For this review, take the finished solid that the model builds, in its own axes (mm). A direction names the side the tool comes from. Coordinates: 2 decimals unless noted, no trailing zeros. Write each loop counter-clockwise with the first axis right and the second up, starting at its lowest first coordinate (ties: lowest second). Pieces come first, ordered by that corner, then holes.
```python
from build123d import *

# Parameters (mm, degrees)
SKETCH2_R           = 1
BOSS_EXTRUDE1_DEPTH = 0.375
CHAMFER1_SIZE       = 0.25
CHAMFER2_SIZE       = 0.5
FILLET1_R           = 0.25


with BuildPart() as part:
    # Sketch1 → Revolve1 (revolve)
    with BuildSketch(Plane.XY):
        with BuildLine():
            Line((-2, 0), (-5.25, 0))
            Line((-5.25, 0), (-5.25, -3))
            Line((-5.25, -3), (-4, -3))
            Line((-4, -3), (-4, -12))
            Line((-4, -12), (-3.34, -12))
            Line((-3.34, -12), (-3.34, -16.5))
            ThreePointArc((-3.34, -16.5), (-3.193553391, -16.853553391), (-2.84, -17))
            Line((-2.84, -17), (-2.5, -17))
            Line((-2.5, -17), (-2.5, -20))
            Line((-2.5, -20), (0, -20))
            Line((0, -20), (0, -8))
            Line((0, -8), (-2, -8))
            Line((-2, -8), (-2, 0))
        make_face()
    revolve(axis=Axis((0, -20, 0), (0, -1, 0)))

    # Sketch2 → Boss-Extrude1 (add, symmetric)
    with BuildSketch(Plane.XY):
        with BuildLine():
            Line((-2.4, -20), (-2.4, -27.8))
            ThreePointArc((-2.4, -27.8), (-2.253553391, -28.153553391), (-1.9, -28.3))
            Line((-1.9, -28.3), (1.9, -28.3))
            ThreePointArc((1.9, -28.3), (2.253553391, -28.153553391), (2.4, -27.8))
            Line((2.4, -27.8), (2.4, -20))
            Line((2.4, -20), (-2.4, -20))
        make_face()
        with Locations((0, -24.15)):
            Circle(SKETCH2_R, mode=Mode.SUBTRACT)
    extrude(amount=BOSS_EXTRUDE1_DEPTH, both=True)

    # Chamfer1
    # the kernel refuses this chamfer: 0.25 mm, written as the material it takes off along each edge
    with BuildSketch(Plane(origin=(0, -20, 0), x_dir=(-1, 0, 0), z_dir=(0, 0, 1))) as chamfer1_piece_1_section:
        Polygon((2.5 - CHAMFER1_SIZE, 0), (2.5, -CHAMFER1_SIZE), (2.5, 0), align=None)
    chamfer1_piece_1 = revolve(axis=Axis((0, -20, 0), (0, -1, 0)), mode=Mode.PRIVATE)
    chamfer1_piece_1 = split(chamfer1_piece_1, bisect_by=Plane(origin=(-2.4, -19.896022541, 0), z_dir=(-1, 0, 0)), keep=Keep.TOP, mode=Mode.PRIVATE)
    add(chamfer1_piece_1, mode=Mode.SUBTRACT)
    with BuildSketch(Plane(origin=(0, -20, 0), x_dir=(-1, 0, 0), z_dir=(0, 0, 1))) as chamfer1_piece_2_section:
        Polygon((2.5 - CHAMFER1_SIZE, 0), (2.5, -CHAMFER1_SIZE), (2.5, 0), align=None)
    chamfer1_piece_2 = revolve(axis=Axis((0, -20, 0), (0, -1, 0)), mode=Mode.PRIVATE)
    chamfer1_piece_2 = split(chamfer1_piece_2, bisect_by=Plane(origin=(-7e-09, -19.879189064, -0.375), z_dir=(0, 0, -1)), keep=Keep.TOP, mode=Mode.PRIVATE)
    add(chamfer1_piece_2, mode=Mode.SUBTRACT)
    with BuildSketch(Plane(origin=(0, -20, 0), x_dir=(-1, 0, 0), z_dir=(0, 0, 1))) as chamfer1_piece_3_section:
        Polygon((2.5 - CHAMFER1_SIZE, 0), (2.5, -CHAMFER1_SIZE), (2.5, 0), align=None)
    chamfer1_piece_3 = revolve(axis=Axis((0, -20, 0), (0, -1, 0)), mode=Mode.PRIVATE)
    chamfer1_piece_3 = split(chamfer1_piece_3, bisect_by=Plane(origin=(-7e-09, -19.879189064, 0.375), z_dir=(0, 0, 1)), keep=Keep.TOP, mode=Mode.PRIVATE)
    add(chamfer1_piece_3, mode=Mode.SUBTRACT)
    with BuildSketch(Plane(origin=(0, -20, 0), x_dir=(-1, 0, 0), z_dir=(0, 0, 1))) as chamfer1_piece_4_section:
        Polygon((2.5 - CHAMFER1_SIZE, 0), (2.5, -CHAMFER1_SIZE), (2.5, 0), align=None)
    chamfer1_piece_4 = revolve(axis=Axis((0, -20, 0), (0, -1, 0)), mode=Mode.PRIVATE)
    chamfer1_piece_4 = split(chamfer1_piece_4, bisect_by=Plane(origin=(2.4, -19.896022542, 0), z_dir=(1, 0, 0)), keep=Keep.TOP, mode=Mode.PRIVATE)
    add(chamfer1_piece_4, mode=Mode.SUBTRACT)

    # Chamfer2
    chamfer2_edges = [part.edges().sort_by_distance(p)[0] for p in [
        (4, -12, 0),
    ]]
    chamfer(chamfer2_edges, length=CHAMFER2_SIZE)

    # Fillet1
    fillet1_edges = [part.edges().sort_by_distance(p)[0] for p in [
        (2, -8, 0),
        (5.25, -3, 0),
        (5.25, 0, 0),
        (2, 0, 0),
    ]]
    fillet(fillet1_edges, radius=FILLET1_R)


solid = part.part
```
Q1. Tool access review of faces 1 (the cylindrical face through (0.867, -7.31, 3.905)), 2 (the flat face through (0, -20, 1)), 3 (the flat face through (0, -8, 0)): name each direction out of +Z, -Z, +X, -X, +Y, -Y from which nothing blocks a thin tool from reaching the whole face with its end or side.
Ans:
face 1: -Y
face 2: +Z, +X, -X, -Y
face 3: +Y
Q2. Draft analysis for pull direction X (two halves, no side actions). For faces 4 (the cylindrical face through (0.54, -18.39, 2.44)), 5 (the cylindrical face through (0, -4, 2)), 6 (the flat face through (1, -23, -0.375)), state which applies: +X half, -X half, draft (parallel to the pull), parting line (faces both ways), or undercut.
Ans:
face 4: parting line
face 5: undercut
face 6: draft
Q3. For probe 1 along Y at (x, z) = (0, -0.2); probe 2 along X at (y, z) = (-5.5, 0); probe 3 along X at (y, z) = (-8.5, 0), list the stretches that pass through material, from the lowest coordinate up.
Ans:
probe 1: y = -28.3 to -25.15, -23.15 to -8
probe 2: x = -4 to -2, 2 to 4
probe 3: x = -4 to 4
Q4. Add section C-C (y = -6). State the section outline as (x, z) points, then the cut area to 3 significant figures.
Ans:
outline: circle Ø8 at (0, 0); hole circle Ø4 at (0, 0)
area: 37.7 mm2
Q5. Add section B-B (y = -14.25). State the section outline as (x, z) points, then the cut area to 3 significant figures.
Ans:
outline: circle Ø6.68 at (0, 0)
area: 35.0 mm2
Q6. Add section A-A (y = -24.15). State the section outline as (x, z) points (3 decimals).
Ans:
outline: (-2.4, -0.375) - (-1, -0.375) - (-1, 0.375) - (-2.4, 0.375) - close; (1, -0.375) - (2.4, -0.375) - (2.4, 0.375) - (1, 0.375) - close
Q7. Clearance check with flat-ended pins moving along their axes: pin 1 Ø2 at (x, z) = (1, 1.5) entering from -Y; pin 2 Ø1.6 at (x, y) = (0, -24.15) entering from +Z; pin 3 Ø5.5 at (x, y) = (-0.5, -26) entering from +Z (3 decimals); pin 4 Ø1.4 at (x, y) = (-0.5, -22) entering from -Z (3 decimals). State where each tip first meets the part, or that it passes through.
Ans:
pin 1: stops at y = -20
pin 2: passes through
pin 3: stops at z = 0.375
pin 4: stops at z = -0.375
